Geometry check sheet. Reference: the model listing, model coordinates, mm. Face numbers are marked on the shaded views. Coordinates: 2 decimals unless noted, no trailing zeros. Order: outer loops, then holes, each group sorted by start corner. A loop starts at its lowest first (then second) coordinate and runs counter-clockwise, first axis right, second up. Notation, with made-up numbers: M 69,-14.75 L 74,-14.75 A17 ccw 74,-4.75 Z; hole C 72.5,-38.75 d7. An arc over 180 degrees is marked long. One line per item, written item: value. Start each with the question number.
1) Sectioned sample at D-D, the plane z = 0.4. State how many separate pieces and enclosed holes the cut face has, then the cut area to 3 significant figures.
2) Sectioned sample at A-A, the plane y = 0. Enter the section's corners in (x, z) (3 decimals).
3) Draft check along X on the marked faces 1 and 2. Enter one of: pulls with the +X half, pulls with the -X half, needs draft (parallel to the pull), parting line crosses it, or undercut.
4) Sectioned sample at B-B, the plane z = 1.05. Enter the section's corners in (x, y) (3 decimals), then the cut area to 3 significant figures.
5) Sectioned sample at C-C, the plane x = 5. Enter the section's corners in (y, z).
6) Thickness scan on L1, parallel to X at y = -0.15, z = 0.45; L2, parallel to Z at x = 3.25, y = -0.05; L3, parallel to X at y = -0.15, z = 0.25. Record the ranges inside material, lowest first. Write a range as from..to.
```python
from build123d import *

# Parameters (mm, degrees)
SKETCH5_R           = 0.225
SKETCH6_R           = 0.225
BOSS_EXTRUDE2_DEPTH = 2


with BuildPart() as part:
    # Sketch1 → Revolve1 (revolve)
    with BuildSketch(Plane.XY):
        Polygon((2.11, 0), (2.222309461, 0.95), (2.882709461, 0.95), (3.001325793, 0.739819784), (4.618674207, 0.739819784), (4.737290539, 0.95), (5.397690539, 0.95), (5.51, 0), align=None)
    revolve(axis=Axis((0, 0, 0), (1, 0, 0)))

    # Sweep4: sweep along a path in Sketch3
    with BuildLine(Plane(origin=(0, 0, 0), x_dir=(1, 0, 0), z_dir=(0, 1, 0))) as sweep4_path:
        Line((0, -0.949999878), (0, -0.762))
        ThreePointArc((0, -0.762), (0.223184633, -0.223184633), (0.762, 0))
        Line((0.762, 0), (2.222309461, 0))
        Line((2.222309461, 0), (5.51, 0))
        Line((5.51, 0), (6.858, 0))
        ThreePointArc((6.858, 0), (7.396815367, -0.223184633), (7.62, -0.762))
        Line((7.62, -0.762), (7.62, -0.949999878))
    # Sketch5 → Sweep4 (sweep)
    with BuildSketch(Plane.XY.offset(0.949999878)):
        Circle(SKETCH5_R)
    sweep(path=sweep4_path.line)

    # Sketch6 → Boss-Extrude2 (add)
    with BuildSketch(Plane.XY.offset(0.949999878)):
        Circle(SKETCH6_R)
        with Locations((7.62, 0)):
            Circle(SKETCH6_R)
    extrude(amount=BOSS_EXTRUDE2_DEPTH)


solid = part.part
```
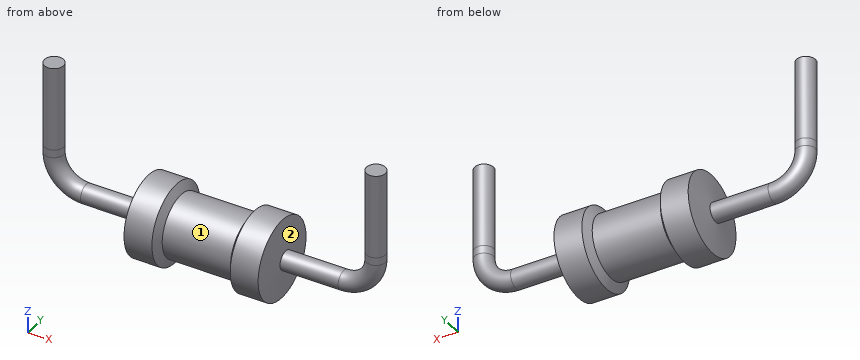
Final values:
1. separate pieces: 3
1. enclosed holes: 0
1. area: 5.15 mm^2
2. outline: M -0.225,0.762 A0.987 ccw 0.762,-0.225 L 2.137,-0.225 L 2.222,-0.95 L 2.883,-0.95 L 3.001,-0.74 L 4.619,-0.74 L 4.737,-0.95 L 5.398,-0.95 L 5.483,-0.225 L 6.858,-0.225 A0.987 ccw 7.845,0.762 L 7.845,2.95 L 7.395,2.95 L 7.395,0.762 A0.537 cw 6.858,0.225 L 5.483,0.225 L 5.398,0.95 L 4.737,0.95 L 4.619,0.74 L 3.001,0.74 L 2.883,0.95 L 2.222,0.95 L 2.137,0.225 L 0.762,0.225 A0.537 cw 0.225,0.762 L 0.225,2.95 L -0.225,2.95 Z
3. face 1: undercut
3. face 2: undercut
4. outline: C 0,0 d0.45; C 7.62,0 d0.45
4. area: 0.318 mm^2
5. outline: C 0,0 d1.9
6. L1: x = -0.11..0.26, 2.17..5.45, 7.36..7.73
6. L2: z = -0.74..0.74
6. L3: x = -0.01..0.46, 2.14..5.48, 7.16..7.63
